Geometry: final body of the model. Coordinates: model frame, mm. Face numbers are marked on the shaded views. Round coordinates to 2 decimals unless told otherwise and drop trailing zeros. Loops run counter-clockwise (first coordinate to the right, second up) from the corner with the lowest first, then second, coordinate; pieces in that order, holes last. Notation, with made-up numbers: (-39.5, 8.25) -> (3.5, 8.25) arc R17 ccw to (3.5, 36.25) -> close; hole circle Ø10 at (-16, 45). An arc over 180 degrees is marked (long way). Answer in a Markdown table with one row per item.
```python
from build123d import *

# Parameters (mm, degrees)
F0_W     = 1228.4
F0_H     = 701.2
F1_DEPTH = 30
F2_W     = 1209.6
F2_H     = 680.4
F3_DEPTH = 2.5


with BuildPart() as f1:
    # F0 (on Top) → F1 (new body)
    with BuildSketch(Plane.XY):
        Rectangle(F0_W, F0_H)
    extrude(amount=F1_DEPTH)

    # F2 (on face) → F3 (cut, symmetric)
    with BuildSketch(Plane(origin=(0, 0, 0), x_dir=(1, 0, 0), z_dir=(0, 0, -1))):
        Rectangle(F2_W, F2_H)
    extrude(amount=-F3_DEPTH, both=True, mode=Mode.SUBTRACT)


solid = f1.part
```
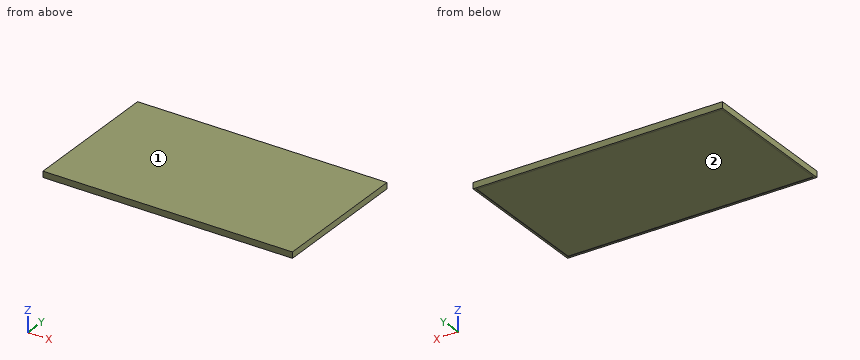
Item 1: Cut plane B-B (y = -240). Output: boundary loops of the cut face in (x, z), then the cut area to 3 significant figures.
Answer:
| item | result |
|---|---|
| outline | (-614.2, 0) -> (-604.8, 0) -> (-604.8, 2.5) -> (604.8, 2.5) -> (604.8, 0) -> (614.2, 0) -> (614.2, 30) -> (-614.2, 30) -> close |
| area | 33,800 mm² |
Item 2: Pin query (flat end, axial travel): pin 1 Ø10 at (x, y) = (89, 209) entering from -Z. Return the tip coordinate at first contact, or that it passes through.
Answer:
| item | result |
|---|---|
| pin 1 | stops at z = 2.5 |
Item 3: Line query: probe 1 along Z at (x, y) = (-282.5, 10.5). Output: solid intervals per line, ascending. Write a range as [from, to].
Answer:
| item | result |
|---|---|
| probe 1 | z = [2.5, 30] |
Item 4: Cut plane A-A (x = 539). Output: boundary loops of the cut face in (y, z).
Answer:
| item | result |
|---|---|
| outline | (-350.6, 0) -> (-340.2, 0) -> (-340.2, 2.5) -> (340.2, 2.5) -> (340.2, 0) -> (350.6, 0) -> (350.6, 30) -> (-350.6, 30) -> close |
Item 5: Draft query along Y for the marked faces 1 and 2. Return one class per face: pulls with the +Y half, pulls with the -Y half, needs draft (parallel to the pull), parting line crosses it, or undercut.
Answer:
| item | result |
|---|---|
| face 1 | needs draft |
| face 2 | undercut |
